For this review, take the finished solid that the model builds, in its own axes (mm). Face numbers are marked on the shaded views. A direction names the side the tool comes from. Coordinates: 2 decimals unless noted, no trailing zeros. Loops run counter-clockwise (first coordinate to the right, second up) from the corner with the lowest first, then second, coordinate; pieces in that order, holes last. Notation, with made-up numbers: (61.25, 6.5) - (93.25, 6.5) arc R17 ccw to (93.25, 36.5) - close; hole circle Ø2 at (-31, 31.5). An arc over 180 degrees is marked (long way). Answer as a JSON object with one key per item and string values. Group by question number.
Item 1: We need section A-A (y = 0.7). State how many separate pieces and enclosed holes the cut face has, then the cut area to 3 significant figures.
Item 2: To check wall thickness, follow line 1 (Z direction, x = 9.25, y = 2.4); line 2 (Z direction, x = -2, y = 4.8); line 3 (Y direction, x = -4.75, z = 1.25). State the ranges of each line that lie inside material, in increasing order.
Item 3: Mouldability with a two-part tool opening along Z and no side actions: class the marked faces 1, 2, 3 and 4 as released by +Z, released by -Z, zero draft, split by the parting line, or undercut.
Item 4: We need section B-B (x = 0.5). Give the boundary of the cut face in (y, z), then the cut area to 3 significant figures.
Item 5: Clearance check with flat-ended pins moving along their axes: pin 1 (1.5 mm diameter, centred on x = 7.5, y = 3, fed in from +Z); pin 2 (2 mm diameter, centred on y = 2.5, z = 3, fed in from -X); pin 3 (2 mm diameter, centred on x = -1.5, y = 3.5, fed in from +Z). State where each tip first meets the part, or that it passes through.
Item 6: Tool access review of the marked faces 5, 6 and 7: name each direction out of +Z, -Z, +X, -X, +Y, -Y from which nothing blocks a thin tool from reaching the whole face with its end or side.
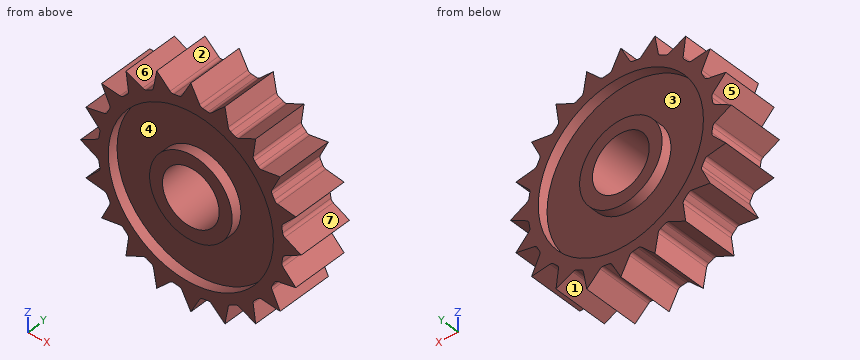
from build123d import *

# Parameters (mm, degrees)
BOSS_EXTRUDE1_DEPTH = 5.5
SKETCH2_R           = 2.75
CUT_EXTRUDE1_DEPTH  = 6.5
SKETCH2_3_R         = 8
SKETCH2_3_R_2       = 4
CUT_EXTRUDE2_DEPTH  = 1
SKETCH3_R           = 8
SKETCH3_R_2         = 4
CUT_EXTRUDE3_DEPTH  = 1


with BuildPart() as part:
    # Sketch1 → Boss-Extrude1 (new body)
    with BuildSketch(Plane(origin=(0, 0, 0), x_dir=(1, 0, 0), z_dir=(0, 1, 0))):
        with BuildLine():
            Line((0, 10.69), (-0.851452759, 9.103207147))
            ThreePointArc((-0.851452759, 9.103207147), (-0.976880558, 8.963010217), (-1.152522076, 8.895650222))
            ThreePointArc((-1.152522076, 8.895650222), (-1.403217151, 8.859564415), (-1.652793464, 8.816415018))
            ThreePointArc((-1.652793464, 8.816415018), (-1.840653858, 8.826201967), (-2.003266017, 8.920777849))
            Line((-2.003266017, 8.920777849), (-3.30339167, 10.166794159))
            Line((-3.30339167, 10.166794159), (-3.622825406, 8.394551104))
            ThreePointArc((-3.622825406, 8.394551104), (-3.698791098, 8.222456579), (-3.845020725, 8.104117202))
            ThreePointArc((-3.845020725, 8.104117202), (-4.072294783, 7.992328522), (-4.296322064, 7.874167684))
            ThreePointArc((-4.296322064, 7.874167684), (-4.478012249, 7.825423572), (-4.661891158, 7.86512066))
            Line((-4.661891158, 7.86512066), (-6.283424347, 8.64839167))
            Line((-6.283424347, 8.64839167), (-6.039570662, 6.864177911))
            ThreePointArc((-6.039570662, 6.864177911), (-6.058638195, 6.677031601), (-6.161141956, 6.519296726))
            ThreePointArc((-6.161141956, 6.519296726), (-6.342747827, 6.342747827), (-6.519296726, 6.161141956))
            ThreePointArc((-6.519296726, 6.161141956), (-6.677031601, 6.058638195), (-6.864177911, 6.039570662))
            Line((-6.864177911, 6.039570662), (-8.64839167, 6.283424347))
            Line((-8.64839167, 6.283424347), (-7.86512066, 4.661891158))
            ThreePointArc((-7.86512066, 4.661891158), (-7.825423572, 4.478012249), (-7.874167684, 4.296322064))
            ThreePointArc((-7.874167684, 4.296322064), (-7.992328522, 4.072294783), (-8.104117202, 3.845020725))
            ThreePointArc((-8.104117202, 3.845020725), (-8.222456579, 3.698791098), (-8.394551104, 3.622825406))
            Line((-8.394551104, 3.622825406), (-10.166794159, 3.30339167))
            Line((-10.166794159, 3.30339167), (-8.920777849, 2.003266017))
            ThreePointArc((-8.920777849, 2.003266017), (-8.826201967, 1.840653858), (-8.816415018, 1.652793464))
            ThreePointArc((-8.816415018, 1.652793464), (-8.859564415, 1.403217151), (-8.895650222, 1.152522076))
            ThreePointArc((-8.895650222, 1.152522076), (-8.963010217, 0.976880558), (-9.103207147, 0.851452759))
            Line((-9.103207147, 0.851452759), (-10.69, 0))
            Line((-10.69, 0), (-9.103207147, -0.851452759))
            ThreePointArc((-9.103207147, -0.851452759), (-8.963010217, -0.976880558), (-8.895650222, -1.152522076))
            ThreePointArc((-8.895650222, -1.152522076), (-8.859564415, -1.403217151), (-8.816415018, -1.652793464))
            ThreePointArc((-8.816415018, -1.652793464), (-8.826201967, -1.840653858), (-8.920777849, -2.003266017))
            Line((-8.920777849, -2.003266017), (-10.166794159, -3.30339167))
            Line((-10.166794159, -3.30339167), (-8.394551104, -3.622825406))
            ThreePointArc((-8.394551104, -3.622825406), (-8.222456579, -3.698791098), (-8.104117202, -3.845020725))
            ThreePointArc((-8.104117202, -3.845020725), (-7.992328522, -4.072294783), (-7.874167684, -4.296322064))
            ThreePointArc((-7.874167684, -4.296322064), (-7.825423572, -4.478012249), (-7.86512066, -4.661891158))
            Line((-7.86512066, -4.661891158), (-8.64839167, -6.283424347))
            Line((-8.64839167, -6.283424347), (-6.864177911, -6.039570662))
            ThreePointArc((-6.864177911, -6.039570662), (-6.677031601, -6.058638195), (-6.519296726, -6.161141956))
            ThreePointArc((-6.519296726, -6.161141956), (-6.342747827, -6.342747827), (-6.161141956, -6.519296726))
            ThreePointArc((-6.161141956, -6.519296726), (-6.058638195, -6.677031601), (-6.039570662, -6.864177911))
            Line((-6.039570662, -6.864177911), (-6.283424347, -8.64839167))
            Line((-6.283424347, -8.64839167), (-4.661891158, -7.86512066))
            ThreePointArc((-4.661891158, -7.86512066), (-4.478012249, -7.825423572), (-4.296322064, -7.874167684))
            ThreePointArc((-4.296322064, -7.874167684), (-4.072294783, -7.992328522), (-3.845020725, -8.104117202))
            ThreePointArc((-3.845020725, -8.104117202), (-3.698791098, -8.222456579), (-3.622825406, -8.394551104))
            Line((-3.622825406, -8.394551104), (-3.30339167, -10.166794159))
            Line((-3.30339167, -10.166794159), (-2.003266017, -8.920777849))
            ThreePointArc((-2.003266017, -8.920777849), (-1.840653858, -8.826201967), (-1.652793464, -8.816415018))
            ThreePointArc((-1.652793464, -8.816415018), (-1.403217151, -8.859564415), (-1.152522076, -8.895650222))
            ThreePointArc((-1.152522076, -8.895650222), (-0.976880558, -8.963010217), (-0.851452759, -9.103207147))
            Line((-0.851452759, -9.103207147), (0, -10.69))
            Line((0, -10.69), (0.851452759, -9.103207147))
            ThreePointArc((0.851452759, -9.103207147), (0.976880558, -8.963010217), (1.152522076, -8.895650222))
            ThreePointArc((1.152522076, -8.895650222), (1.403217151, -8.859564415), (1.652793464, -8.816415018))
            ThreePointArc((1.652793464, -8.816415018), (1.840653858, -8.826201967), (2.003266017, -8.920777849))
            Line((2.003266017, -8.920777849), (3.30339167, -10.166794159))
            Line((3.30339167, -10.166794159), (3.622825406, -8.394551104))
            ThreePointArc((3.622825406, -8.394551104), (3.698791098, -8.222456579), (3.845020725, -8.104117202))
            ThreePointArc((3.845020725, -8.104117202), (4.072294783, -7.992328522), (4.296322064, -7.874167684))
            ThreePointArc((4.296322064, -7.874167684), (4.478012249, -7.825423572), (4.661891158, -7.86512066))
            Line((4.661891158, -7.86512066), (6.283424347, -8.64839167))
            Line((6.283424347, -8.64839167), (6.039570662, -6.864177911))
            ThreePointArc((6.039570662, -6.864177911), (6.058638195, -6.677031601), (6.161141956, -6.519296726))
            ThreePointArc((6.161141956, -6.519296726), (6.342747827, -6.342747827), (6.519296726, -6.161141956))
            ThreePointArc((6.519296726, -6.161141956), (6.677031601, -6.058638195), (6.864177911, -6.039570662))
            Line((6.864177911, -6.039570662), (8.64839167, -6.283424347))
            Line((8.64839167, -6.283424347), (7.86512066, -4.661891158))
            ThreePointArc((7.86512066, -4.661891158), (7.825423572, -4.478012249), (7.874167684, -4.296322064))
            ThreePointArc((7.874167684, -4.296322064), (7.992328522, -4.072294783), (8.104117202, -3.845020725))
            ThreePointArc((8.104117202, -3.845020725), (8.222456579, -3.698791098), (8.394551104, -3.622825406))
            Line((8.394551104, -3.622825406), (10.166794159, -3.30339167))
            Line((10.166794159, -3.30339167), (8.920777849, -2.003266017))
            ThreePointArc((8.920777849, -2.003266017), (8.826201967, -1.840653858), (8.816415018, -1.652793464))
            ThreePointArc((8.816415018, -1.652793464), (8.859564415, -1.403217151), (8.895650222, -1.152522076))
            ThreePointArc((8.895650222, -1.152522076), (8.963010217, -0.976880558), (9.103207147, -0.851452759))
            Line((9.103207147, -0.851452759), (10.69, 0))
            Line((10.69, 0), (9.103207147, 0.851452759))
            ThreePointArc((9.103207147, 0.851452759), (8.963010217, 0.976880558), (8.895650222, 1.152522076))
            ThreePointArc((8.895650222, 1.152522076), (8.859564415, 1.403217151), (8.816415018, 1.652793464))
            ThreePointArc((8.816415018, 1.652793464), (8.826201967, 1.840653858), (8.920777849, 2.003266017))
            Line((8.920777849, 2.003266017), (10.166794159, 3.30339167))
            Line((10.166794159, 3.30339167), (8.394551104, 3.622825406))
            ThreePointArc((8.394551104, 3.622825406), (8.222456579, 3.698791098), (8.104117202, 3.845020725))
            ThreePointArc((8.104117202, 3.845020725), (7.992328522, 4.072294783), (7.874167684, 4.296322064))
            ThreePointArc((7.874167684, 4.296322064), (7.825423572, 4.478012249), (7.86512066, 4.661891158))
            Line((7.86512066, 4.661891158), (8.64839167, 6.283424347))
            Line((8.64839167, 6.283424347), (6.864177911, 6.039570662))
            ThreePointArc((6.864177911, 6.039570662), (6.677031601, 6.058638195), (6.519296726, 6.161141956))
            ThreePointArc((6.519296726, 6.161141956), (6.342747827, 6.342747827), (6.161141956, 6.519296726))
            ThreePointArc((6.161141956, 6.519296726), (6.058638195, 6.677031601), (6.039570662, 6.864177911))
            Line((6.039570662, 6.864177911), (6.283424347, 8.64839167))
            Line((6.283424347, 8.64839167), (4.661891158, 7.86512066))
            ThreePointArc((4.661891158, 7.86512066), (4.478012249, 7.825423572), (4.296322064, 7.874167684))
            ThreePointArc((4.296322064, 7.874167684), (4.072294783, 7.992328522), (3.845020725, 8.104117202))
            ThreePointArc((3.845020725, 8.104117202), (3.698791098, 8.222456579), (3.622825406, 8.394551104))
            Line((3.622825406, 8.394551104), (3.30339167, 10.166794159))
            Line((3.30339167, 10.166794159), (2.003266017, 8.920777849))
            ThreePointArc((2.003266017, 8.920777849), (1.840653858, 8.826201967), (1.652793464, 8.816415018))
            ThreePointArc((1.652793464, 8.816415018), (1.403217151, 8.859564415), (1.152522076, 8.895650222))
            ThreePointArc((1.152522076, 8.895650222), (0.976880558, 8.963010217), (0.851452759, 9.103207147))
            Line((0.851452759, 9.103207147), (0, 10.69))
        make_face()
    extrude(amount=BOSS_EXTRUDE1_DEPTH)

    # Sketch2 → Cut-Extrude1 (cut, through all)
    with BuildSketch(Plane(origin=(0, 5.5, 0), x_dir=(1, 0, 0), z_dir=(0, 1, 0))):
        Circle(SKETCH2_R)
    extrude(amount=-CUT_EXTRUDE1_DEPTH, mode=Mode.SUBTRACT)

    # Sketch2_3 → Cut-Extrude2 (cut)
    with BuildSketch(Plane(origin=(0, 5.5, 0), x_dir=(1, 0, 0), z_dir=(0, 1, 0))):
        Circle(SKETCH2_3_R)
        Circle(SKETCH2_3_R_2, mode=Mode.SUBTRACT)
    extrude(amount=-CUT_EXTRUDE2_DEPTH, mode=Mode.SUBTRACT)

    # Sketch3 → Cut-Extrude3 (cut)
    with BuildSketch(Plane.XZ):
        Circle(SKETCH3_R)
        Circle(SKETCH3_R_2, mode=Mode.SUBTRACT)
    extrude(amount=-CUT_EXTRUDE3_DEPTH, mode=Mode.SUBTRACT)


solid = part.part
Check sheet entries:
{
 "1": {"separate pieces": "2", "enclosed holes": "2", "area": "111 mm2"},
 "2": {"line 1": "z = -3.47 to -2.35, -0.77 to 0.77, 2.35 to 3.47", "line 2": "z = -8.92 to -7.75, -3.46 to -1.89, 1.89 to 3.46, 7.75 to 8.92", "line 3": "y = 1 to 4.5"},
 "3": {"face 1": "released by -Z", "face 2": "released by +Z", "face 3": "undercut", "face 4": "undercut"},
 "4": {"outline": "(0, -9.76) - (5.5, -9.76) - (5.5, -7.98) - (4.5, -7.98) - (4.5, -3.97) - (5.5, -3.97) - (5.5, -2.7) - (0, -2.7) - (0, -3.97) - (1, -3.97) - (1, -7.98) - (0, -7.98) - close; (0, 2.7) - (5.5, 2.7) - (5.5, 3.97) - (4.5, 3.97) - (4.5, 7.98) - (5.5, 7.98) - (5.5, 9.76) - (0, 9.76) - (0, 7.98) - (1, 7.98) - (1, 3.97) - (0, 3.97) - close", "area": "61.5 mm2"},
 "5": {"pin 1": "stops at z = 6.23", "pin 2": "stops at x = -10.17", "pin 3": "stops at z = 9.76"},
 "6": {"face 5": "-X, +Y, -Y", "face 6": "+Z, +Y, -Y", "face 7": "+X, +Y, -Y"}
}
